Check sheet for the modelled part. Datum: model origin and axes. Units: mm. Face numbers are marked on the shaded views. A direction names the side the tool comes from. Give positions to 0.01 mm unless a question says otherwise; leave off trailing zeros. Write each loop counter-clockwise with the first axis right and the second up, starting at its lowest first coordinate (ties: lowest second). Pieces come first, ordered by that corner, then holes. Notation, with made-up numbers: (35.25, -6) -> (68.25, -6) arc R21 cw to (68.25, 33) -> close; hole circle Ø1 at (7, 73.25). An arc over 180 degrees is marked (long way). Answer as a JSON object with one key per item and string values.
from build123d import *

# Parameters (mm, degrees)
SKETCH1_W           = 71
SKETCH1_H           = 25.5
BOSS_EXTRUDE2_DEPTH = 4
SKETCH4_W           = 7
SKETCH4_H           = 16
BOSS_EXTRUDE3_DEPTH = 8
SKETCH5_W           = 19.05
SKETCH5_H           = 19.05
BOSS_EXTRUDE4_DEPTH = 3.174
SKETCH6_R           = 1.5
CUT_EXTRUDE1_DEPTH  = 5


with BuildPart() as part:
    # Sketch1 → Boss-Extrude2 (new body)
    with BuildSketch(Plane(origin=(0, 0, 0), x_dir=(1, 0, 0), z_dir=(0, 1, 0))):
        Rectangle(SKETCH1_W, SKETCH1_H)
    extrude(amount=BOSS_EXTRUDE2_DEPTH)

    # Sketch4 → Boss-Extrude3 (add)
    with BuildSketch(Plane(origin=(0, 4, 0), x_dir=(1, 0, 0), z_dir=(0, 1, 0))):
        with Locations((32, 0)):
            Rectangle(SKETCH4_W, SKETCH4_H)
    extrude(amount=BOSS_EXTRUDE3_DEPTH)

    # Sketch5 → Boss-Extrude4 (add)
    with BuildSketch(Plane(origin=(0, 4, 0), x_dir=(1, 0, 0), z_dir=(0, 1, 0))):
        Rectangle(SKETCH5_W, SKETCH5_H)
    extrude(amount=BOSS_EXTRUDE4_DEPTH)

    # Sketch6 → Cut-Extrude1 (cut, through all)
    with BuildSketch(Plane(origin=(0, 4, 0), x_dir=(1, 0, 0), z_dir=(0, 1, 0))):
        with Locations((-31.302, 9.525)):
            Circle(SKETCH6_R)
        with Locations((-31.302, -9.525)):
            Circle(SKETCH6_R)
        with Locations((25.848, 9.525)):
            Circle(SKETCH6_R)
        with Locations((25.848, -9.525)):
            Circle(SKETCH6_R)
    extrude(amount=-CUT_EXTRUDE1_DEPTH, mode=Mode.SUBTRACT)


solid = part.part
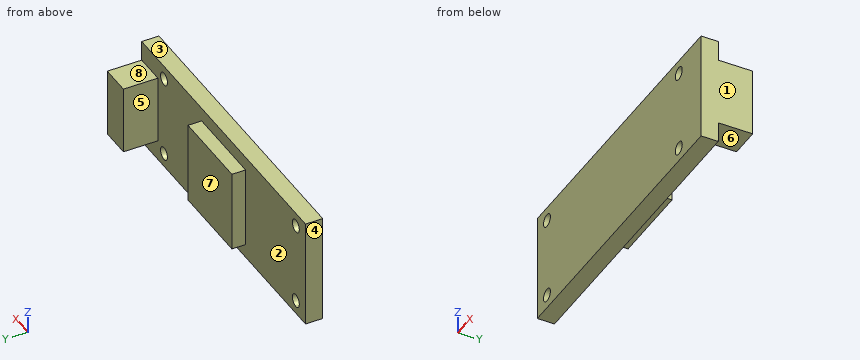
1. Sectioned sample at A-A, the plane y = 6. Enter the section's corners in (x, z) (3 decimals), plus the area to 3 significant figures.
Determined:
{"outline": "(-9.525, -9.525) -> (9.525, -9.525) -> (9.525, 9.525) -> (-9.525, 9.525) -> close; (28.5, -8) -> (35.5, -8) -> (35.5, 8) -> (28.5, 8) -> close", "area": "475 mm^2"}
2. Mould release check, pull along X, two halves, no side actions. Record for the marked faces 1, 2, 3 and 4: released by +X, released by -X, zero draft, split by the parting line, or undercut.
Determined:
{"face 1": "released by +X", "face 2": "undercut", "face 3": "zero draft", "face 4": "released by -X"}
3. Go/stop test with flat-tipped pins: P1, Ø7.5, axis at x = 12.5, z = 2, coming from the +Y side; P2, Ø12, axis at x = -26, z = 6.5, coming from the +Y side; P3, Ø1.5, axis at y = 8, z = 2.5, coming from the -X side; P4, Ø1.8, axis at x = -31.302, z = 9.525, coming from the +Y side. Record where each tip stops, or that it passes through.
Determined:
{"P1": "y = 7.17", "P2": "y = 4", "P3": "x = 28.5", "P4": "through"}
4. Sectioned sample at D-D, the plane z = -3.75. Enter the section's corners in (x, y) (3 decimals).
Determined:
{"outline": "(-35.5, 0) -> (35.5, 0) -> (35.5, 12) -> (28.5, 12) -> (28.5, 4) -> (9.525, 4) -> (9.525, 7.174) -> (-9.525, 7.174) -> (-9.525, 4) -> (-35.5, 4) -> close"}
5. Sectioned sample at B-B, the plane x = 5.5. Enter the section's corners in (y, z) (3 decimals).
Determined:
{"outline": "(0, -12.75) -> (4, -12.75) -> (4, -9.525) -> (7.174, -9.525) -> (7.174, 9.525) -> (4, 9.525) -> (4, 12.75) -> (0, 12.75) -> close"}
6. Scan lines: L1, parallel to X at y = 6.75, z = -2.75 (3 decimals); L2, parallel to Z at x = -1.5, y = 7 (3 decimals); L3, parallel to X at y = 11.25, z = -2.75. Record each from-to range of solid material in increasing order. Write a range as [from, to].
Determined:
{"L1": "[-9.525, 9.525], [28.5, 35.5]", "L2": "[-9.525, 9.525]", "L3": "[28.5, 35.5]"}
7. Sectioned sample at C-C, the plane y = 3.25. Enter the section's corners in (x, z) (3 decimals).
Determined:
{"outline": "(-35.5, -12.75) -> (35.5, -12.75) -> (35.5, 12.75) -> (-35.5, 12.75) -> close; hole circle Ø3 at (-31.302, -9.525); hole circle Ø3 at (-31.302, 9.525); hole circle Ø3 at (25.848, -9.525); hole circle Ø3 at (25.848, 9.525)"}
8. Access from +Z, -Z, +X, -X, +Y, -Y to the whole of each face (thin tool, end or side, straight path). Record for the marked faces 5, 6, 7 and 8.
Determined:
{"face 5": "+Z, -Z, +Y", "face 6": "-Z, +X, +Y", "face 7": "+Z, -Z, -X, +Y", "face 8": "+Z, +X, +Y"}
